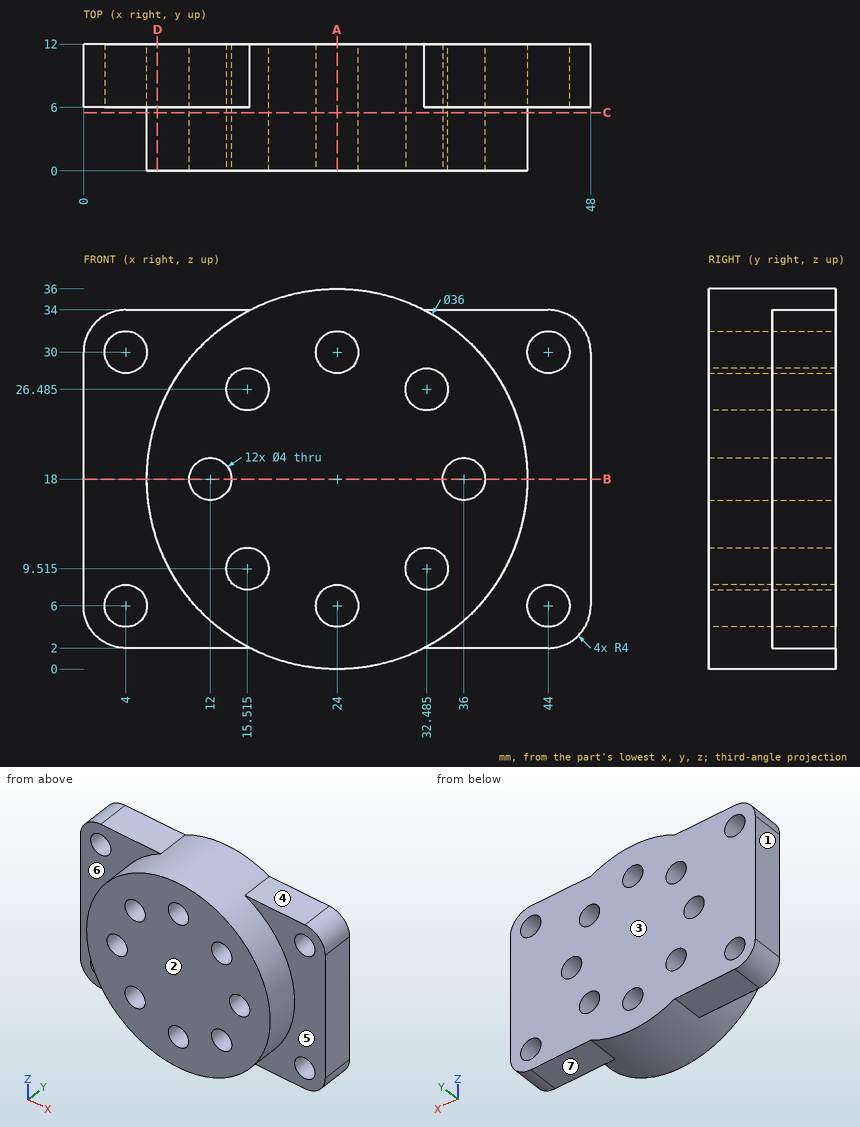
The drawing under review shows one solid part. Ordinate dimensions are in mm from its lowest x, y, z. A direction names the side the tool comes from. Round coordinates to 2 decimals unless told otherwise and drop trailing zeros. Write each loop counter-clockwise with the first axis right and the second up, starting at its lowest first coordinate (ties: lowest second). Pieces come first, ordered by that corner, then holes. Notation, with made-up numbers: (46, -11.5) - (71, -11.5) arc R22 ccw to (71, -0.5) - close; hole circle Ø9 at (-27, 83.25). An arc over 180 degrees is marked (long way). Use a Markdown table: item, result. Add a question column.
1. We need section B-B (z = 18). State the section outline as (x, y) points.
2. We need section D-D (x = 7). State the section outline as (y, z) points, then the cut area to 3 significant figures.
3. Wall thickness on probe 1 along Z at (x, y) = (4, 9.75); probe 2 along X at (y, z) = (7.75, 18); probe 3 along X at (y, z) = (9.5, 9): over which ranges is each line inside the solid? List them lowest first.
4. Mouldability with a two-part tool opening along Y and no side actions: class the marked faces 1, 2 and 3 as +Y half, -Y half, draft (parallel to the pull), parting line (faces both ways), or undercut.
5. Clearance check with flat-ended pins moving along their axes: pin 1 (3.5 mm diameter, centred on x = 24, z = 30, fed in from +Y); pin 2 (3 mm diameter, centred on x = 35.5, y = 9.5, fed in from -Z); pin 3 (5 mm diameter, centred on x = 39, y = 8, fed in from +Z); pin 4 (2 mm diameter, centred on x = 22, y = 10, fed in from -Z). State where each tip first meets the part, or that it passes through.
6. We need section C-C (y = 5.5). Count the separate pieces of the cut face and the enclosed holes in it, then the cut area to 3 significant figures.
7. For the marked faces 4, 5, 6 and 7, list the 3-axis set-ups (+Z, -Z, +X, -X, +Y, -Y) from which the entire face can be reached by the end or side of a thin tool; tool diameter is ignored.
8. We need section A-A (x = 24). State the section outline as (y, z) points, then the cut area to 3 significant figures.
Output:
| question | item | result |
|---|---|---|
| 1 | outline | (0, 6) - (6, 6) - (6, 0) - (10, 0) - (10, 12) - (0, 12) - close; (14, 0) - (34, 0) - (34, 12) - (14, 12) - close; (38, 0) - (42, 0) - (42, 6) - (48, 6) - (48, 12) - (38, 12) - close |
| 2 | outline | (0, 12.08) - (6, 12.08) - (6, 2) - (12, 2) - (12, 34) - (6, 34) - (6, 23.92) - (0, 23.92) - close |
| 2 | area | 263 mm2 |
| 3 | probe 1 | z = 2 to 4, 8 to 28, 32 to 34 |
| 3 | probe 2 | x = 0 to 10, 14 to 34, 38 to 48 |
| 3 | probe 3 | x = 0 to 13.58, 17.45 to 30.55, 34.42 to 48 |
| 4 | face 1 | draft |
| 4 | face 2 | -Y half |
| 4 | face 3 | +Y half |
| 5 | pin 1 | passes through |
| 5 | pin 2 | stops at z = 2 |
| 5 | pin 3 | stops at z = 34 |
| 5 | pin 4 | stops at z = 0.03 |
| 6 | separate pieces | 1 |
| 6 | enclosed holes | 8 |
| 6 | area | 917 mm2 |
| 7 | face 4 | +Z, +X, +Y, -Y |
| 7 | face 5 | +X, -Y |
| 7 | face 6 | -X, -Y |
| 7 | face 7 | -Z, +X, +Y, -Y |
| 8 | outline | (0, 0) - (12, 0) - (12, 4) - (0, 4) - close; (0, 8) - (12, 8) - (12, 28) - (0, 28) - close; (0, 32) - (12, 32) - (12, 36) - (0, 36) - close |
| 8 | area | 336 mm2 |
